Source: CAD feature listing. Evaluate the final solid. Frame: model axes, mm. Face numbers are marked on the shaded views. A direction names the side the tool comes from. Round coordinates to 2 decimals unless told otherwise and drop trailing zeros. Loops run counter-clockwise (first coordinate to the right, second up) from the corner with the lowest first, then second, coordinate; pieces in that order, holes last.
Item 1: Section query B-B on y = 5.75. Return loops of the section in (x, z), then the cut area to 3 significant figures.
Item 2: Ray query, L1, parallel to X at y = 11.75, z = 0; L2, parallel to Z at x = 0.25, y = 5.75; L3, parallel to Z at x = 1, y = -1.75. Return the intervals inside material, ascending.
Item 3: First-contact query: P1, Ø1.2, axis at y = 7.5, z = 0, coming from the -X side; P2, Ø0.8, axis at x = 1, y = 8, coming from the -Z side; P3, Ø5, axis at y = 1.5, z = -4, coming from the +X side. Flat tips, straight axial feed; report the tip coordinate or a pass-through.
Item 4: Pull-direction query (Y, two-part tool) for the marked faces 1, 2 and 3; classes: released by +Y, released by -Y, zero draft, split by the parting line, or undercut.
Item 5: Section query D-D on z = 2.25. Return loops of the section in (x, y).
Item 6: Section query C-C on y = -0.75. Return loops of the section in (x, z), then the cut area to 3 significant figures.
Item 7: Access query for the marked faces 4 and 5. Directions: +Z, -Z, +X, -X, +Y, -Y. A direction counts if a zero-diameter tool reaches every point of the face in a straight line with its end or side. Return the directions, or none.
```python
from build123d import *

# Parameters (mm, degrees)
SKETCH1_W               = 7.5
SKETCH1_H               = 15
CUT_EXTRUDE1_START      = -20
CUT_EXTRUDE1_DEPTH      = 20
SKETCH4_W               = 1.5
SKETCH4_H               = 1.5
CUT_EXTRUDE2_DEPTH      = 20
CUT_EXTRUDE3_DEPTH      = 17.075914552
CUT_EXTRUDE3_DEPTH_BACK = 17.075914552
CUT_EXTRUDE4_DEPTH      = 17.075914721
CUT_EXTRUDE4_DEPTH_BACK = 17.075914721
SKETCH8_W               = 12.380653288
SKETCH8_H               = 7.175906378
CUT_EXTRUDE5_DEPTH      = 0.5
FILLET2_R               = 1
FILLET5_R               = 0.5


with BuildPart() as part:
    # Sketch1 → Revolve1 (revolve)
    with BuildSketch(Plane.XY):
        with Locations((-3.75, 4.580357143)):
            Rectangle(SKETCH1_W, SKETCH1_H)
    revolve(axis=Axis((0, 12.080357143, 0), (0, -1, 0)))

    # Sketch2 → Cut-Extrude1 (cut)
    with BuildSketch(Plane.XZ.offset(2.919642857).offset(CUT_EXTRUDE1_START)):
        with BuildLine():
            Line((-3.5, 6.633249581), (-3.5, -6.633249581))
            ThreePointArc((-3.5, -6.633249581), (-7.5, 0), (-3.5, 6.633249581))
        make_face()
    extrude(amount=CUT_EXTRUDE1_DEPTH, mode=Mode.SUBTRACT)

    # Sketch4 → Cut-Extrude2 (cut)
    with BuildSketch(Plane.XZ.offset(2.919642857)):
        with Locations((0.588025285, -0.043999564)):
            Rectangle(SKETCH4_W, SKETCH4_H)
    extrude(amount=-CUT_EXTRUDE2_DEPTH, mode=Mode.SUBTRACT)

    # Sketch6 → Cut-Extrude3 (cut, two sides: drawn at the far end of the back side and taken through both)
    with BuildSketch(Plane.XY.offset(-CUT_EXTRUDE3_DEPTH_BACK)):
        with BuildLine():
            Line((2.684394406, 0.589840789), (5.221333223, 0.589840789))
            ThreePointArc((5.221333223, 0.589840789), (6.01349632, -0.202322309), (5.221333223, -0.994485407))
            Line((5.221333223, -0.994485407), (5.524196013, -2.919642857))
            Line((5.524196013, -2.919642857), (3.217926739, -2.919642857))
            Line((3.217926739, -2.919642857), (2.84197746, -0.994485407))
            ThreePointArc((2.84197746, -0.994485407), (2.755326831, -1.007008376), (2.667826658, -1.009987637))
            ThreePointArc((2.667826658, -1.009987637), (1.8844373, -0.201874894), (2.684394406, 0.589840789))
        make_face()
        with BuildLine():
            Line((2.84197746, 8.328542626), (5.04197746, 8.328542626))
            ThreePointArc((5.04197746, 8.328542626), (5.761372587, 8.781718764), (5.663273755, 9.626274613))
            ThreePointArc((5.663273755, 9.626274613), (5.448979722, 9.81206297), (5.183221531, 9.91111765))
            Line((5.183221531, 9.91111765), (4.385819176, 12.080357143))
            Line((4.385819176, 12.080357143), (1.90930103, 12.080357143))
            Line((1.90930103, 12.080357143), (2.840116682, 9.928540462))
            ThreePointArc((2.840116682, 9.928540462), (2.515101589, 9.858715321), (2.24652895, 9.662809481))
            ThreePointArc((2.24652895, 9.662809481), (2.111425106, 8.802516157), (2.84197746, 8.328542626))
        make_face()
    extrude(amount=CUT_EXTRUDE3_DEPTH + CUT_EXTRUDE3_DEPTH_BACK, mode=Mode.SUBTRACT)

    # Sketch7 → Cut-Extrude4 (cut, two sides: drawn at the far end of the back side and taken through both)
    with BuildSketch(Plane.XY.offset(-CUT_EXTRUDE4_DEPTH_BACK)):
        Polygon((-3.5, 0.600357143), (-3.5, -2.919642857), (-1, -2.919642857), align=None)
        Polygon((-3.5, 12.080357143), (-3.5, 8.580357143), (-1, 12.080357143), align=None)
    extrude(amount=CUT_EXTRUDE4_DEPTH + CUT_EXTRUDE4_DEPTH_BACK, mode=Mode.SUBTRACT)

    # Sketch8 → Cut-Extrude5 (cut)
    with BuildSketch(Plane.ZY.offset(3.5)):
        with Locations((-0.033221789, 4.583246246)):
            Rectangle(SKETCH8_W, SKETCH8_H)
    extrude(amount=-CUT_EXTRUDE5_DEPTH, mode=Mode.SUBTRACT)

    # Fillet2
    fillet2_edges = [part.edges().sort_by_distance(p)[0] for p in [
        (-1, 12.080357143, 0),
        (-3.5, 8.580357143, 0),
        (-1, -2.919642857, 0),
        (-3.5, 0.600357143, 0),
    ]]
    fillet(fillet2_edges, radius=FILLET2_R)

    # Fillet5
    # the kernel refuses this fillet: 0.5 mm, written as the material it takes off along each edge
    with BuildSketch(Plane(origin=(-3.5, 8.171199435, 6.157104855), x_dir=(0, 0, 1), z_dir=(0, -1, 0)), Plane(origin=(-3.5, 0.995293057, -6.223548433), x_dir=(0, 0, -1), z_dir=(0, 1, 0))) as fillet5_piece_1:
        with BuildLine():
            CenterArc((FILLET5_R, -FILLET5_R), FILLET5_R, 90, 90)
            Line((0, -FILLET5_R), (0, 0))
            Line((0, 0), (FILLET5_R, 0))
        make_face()
    extrude(amount=7.175906378, mode=Mode.SUBTRACT)


solid = part.part
```
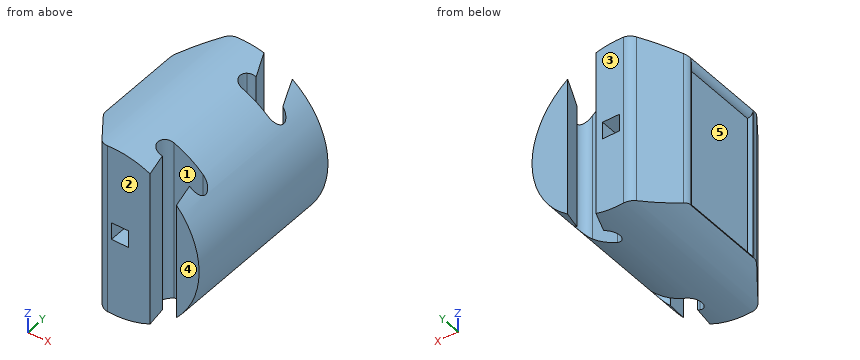
Data:
1. outline: (-3.5, 6.63) arc R0.5 ccw to (-3, 6.16) - (-3, -6.22) arc R0.5 ccw to (-3.49, -6.64) arc R7.5 ccw (long way) to start; hole (-0.16, -0.79) - (1.34, -0.79) - (1.34, 0.71) - (-0.16, 0.71) - close
1. area: 130 mm2
2. L1: x = -1.23 to -0.16, 1.34 to 2.05, 4.51 to 7.5
2. L2: z = -7.5 to -0.79, 0.71 to 7.5
2. L3: z = -7.43 to -0.79, 0.71 to 7.43
3. P1: stops at x = -3
3. P2: stops at z = -7.48
3. P3: stops at x = 7.35
4. face 1: undercut
4. face 2: released by -Y
4. face 3: released by +Y
5. outline: (-3.5, 0.92) arc R1 ccw to (-3.32, 0.34) - (-1.3, -2.5) arc R1 ccw to (-0.48, -2.92) - (3.22, -2.92) - (2.84, -0.99) arc R0.8 cw (long way) to (2.68, 0.59) - (5.22, 0.59) arc R0.79 cw to (5.22, -0.99) - (5.52, -2.92) - (7.15, -2.92) - (7.15, 12.08) - (4.39, 12.08) - (5.18, 9.91) arc R0.8 cw to (5.04, 8.33) - (2.84, 8.33) arc R0.8 cw to (2.84, 9.93) - (1.91, 12.08) - (-0.49, 12.08) arc R1 ccw to (-1.3, 11.66) - (-3.31, 8.84) arc R1 ccw to (-3.5, 8.26) - (-3.5, 8.17) - (-3, 8.17) - (-3, 1) - (-3.5, 1) - close
6. outline: (-2.54, -7.06) arc R7.5 ccw to (2.09, -7.2) - (2.09, 7.2) arc R7.5 ccw to (-2.54, 7.06) - close; (5.79, -4.76) arc R7.5 ccw to (5.79, 4.76) - close; hole (-0.16, -0.79) - (1.34, -0.79) - (1.34, 0.71) - (-0.16, 0.71) - close
6. area: 77.2 mm2
7. face 4: +Z, -Z, +X, -X, -Y
7. face 5: -X
